```python
from build123d import *

# Parameters (mm, degrees)
SKETCH_W     = 254
SKETCH_H     = 17
PAD_DEPTH    = 5
SKETCH001_W  = 250
SKETCH001_H  = 2
POCKET_DEPTH = 15
FILLET_R     = 2.49


with BuildPart() as part:
    # Sketch → Pad (new body)
    with BuildSketch(Plane.XY):
        Rectangle(SKETCH_W, SKETCH_H)
    extrude(amount=PAD_DEPTH)

    # Sketch001 (on Face2 of Pad) → Pocket (cut)
    with BuildSketch(Plane.XZ.offset(8.5)):
        with Locations((0, 2.5)):
            Rectangle(SKETCH001_W, SKETCH001_H)
    extrude(amount=-POCKET_DEPTH, mode=Mode.SUBTRACT)

    # Fillet
    fillet_edges = [part.edges().sort_by_distance(p)[0] for p in [
        (127, 0, 5),
        (127, 0, 0),
        (-127, 0, 0),
        (-127, 0, 5),
    ]]
    fillet(fillet_edges, radius=FILLET_R)


solid = part.part
```
Design review of the part built by this model. Coordinates are the model's own, in mm. A direction names the side the tool comes from. Round coordinates to 2 decimals unless told otherwise and drop trailing zeros. Write each loop counter-clockwise with the first axis right and the second up, starting at its lowest first coordinate (ties: lowest second). Pieces come first, ordered by that corner, then holes. Notation, with made-up numbers: (32.25, 82.25) -> (91.25, 82.25) arc R30 ccw to (91.25, 120.25) -> close; hole circle Ø7 at (74, 28.25). An arc over 180 degrees is marked (long way). Write item = value, one per line. Start each with the question number.
1) Clearance check with a flat-ended pin moving along its axis: pin 1 (2 mm diameter, centred on y = -2.5, z = 4.5, fed in from +X). State where the tip first meets the part, or that it passes through.
2) Mouldability with a two-part tool opening along Z and no side actions: class faces 1 (the face through (-2, 0, 5)), 2 (the face through (-2, 8.5, 2)), 3 (the face through (-2, 0, 0)), 4 (the face through (-2, -1, 3.5)) as +Z half, -Z half, draft (parallel to the pull), parting line (faces both ways), or undercut.
3) Wall thickness on probe 1 along X at (y, z) = (5, 2.05); probe 2 along Z at (x, y) = (-42, -7); probe 3 along Y at (x, z) = (-70, 2.25): over which ranges is each line inside the solid? List them lowest first. Write a range as from..to.
4) Take a section at B-B, the plane x = -63. State the section outline as (y, z) points.
5) Tool access review of faces 5 (the face through (-2, -1, 1.5)), 6 (the face through (-2, -8.5, 1)): name each direction out of +Z, -Z, +X, -X, +Y, -Y from which nothing blocks a thin tool from reaching the whole face with its end or side.
Results list:
q1.pin_1 = 126.79
q2.face_1 = +Z half
q2.face_2 = draft
q2.face_3 = -Z half
q2.face_4 = undercut
q3.probe_1 = -126.96..-125, 125..126.96
q3.probe_2 = 0..1.5, 3.5..5
q3.probe_3 = 6.5..8.5
q4.outline = (-8.5, 0) -> (8.5, 0) -> (8.5, 5) -> (-8.5, 5) -> (-8.5, 3.5) -> (6.5, 3.5) -> (6.5, 1.5) -> (-8.5, 1.5) -> close
q5.face_5 = -Y
q5.face_6 = +Z, -Z, +X, -X, -Y
